from build123d import *

# Parameters (mm, degrees)
F0_W     = 100
F0_H     = 150
F1_DEPTH = 47
F2_R     = 33.5
F3_DEPTH = 22
F4_R     = 5
F5_DEPTH = 12


with BuildPart() as f1:
    # F0 (on Front) → F1 (new body)
    with BuildSketch(Plane.XZ):
        Rectangle(F0_W, F0_H)
    extrude(amount=F1_DEPTH)

    # F2 (on face) → F3 (join)
    with BuildSketch(Plane.XZ.offset(47)):
        with Locations((0, 30)):
            Circle(F2_R)
    extrude(amount=F3_DEPTH)

    # F4 (on face) → F5 (cut)
    with BuildSketch(Plane.XZ.offset(47)):
        with Locations((50, -17)):
            Circle(F4_R)
        with Locations((-50, -17)):
            Circle(F4_R)
    extrude(amount=-F5_DEPTH, mode=Mode.SUBTRACT)


solid = f1.part
The listing builds one solid part. Answer for the finished solid, in the listing's coordinates (mm). A direction names the side the tool comes from. Coordinates: 2 decimals unless noted, no trailing zeros. Write each loop counter-clockwise with the first axis right and the second up, starting at its lowest first coordinate (ties: lowest second). Pieces come first, ordered by that corner, then holes. Notation, with made-up numbers: M 78,63 L 97,63 A21 cw 97,85 Z; hole C 53.25,89.25 d6. An arc over 180 degrees is marked long. Use one line per item in the form item = value.
Item 1: Find section C-C, the plane y = -55.5. Give the vertices of the cut face in (x, z).
Model answer:
outline = C 0,30 d67
Item 2: Given P1, Ø1.5, axis at x = 46.5, z = -17.5, coming from the -Y side; P2, Ø4, axis at x = 31.5, z = -11.5, coming from the -Y side; P3, Ø10, axis at x = 34, z = -54.5, coming from the +Y side, each flat-ended and moving along its own axis, determine where each tip first touches the part or whether it passes through.
Model answer:
P1 = -35
P2 = -47
P3 = 0
Item 3: Find section A-A, the plane z = -17. Give the vertices of the cut face in (x, y), plus the area to 3 significant figures.
Model answer:
outline = M -50,-35 L -45,-35 L -45,-47 L 45,-47 L 45,-35 L 50,-35 L 50,0 L -50,0 Z
area = 4,580 mm2
Item 4: For faces 4 (the face through (48, -35, -17)), 5 (the face through (-45, -41, -17)), 6 (the face through (0, -69, 30)), 7 (the face through (50, -23, -1)), 8 (the face through (31.953, -57.846, 40.062)), determine the directions among +Z, -Z, +X, -X, +Y, -Y from which every point of the face is accessible in a straight line to the end or side of a thin tool.
Model answer:
face_4 = +X, -Y
face_5 = -X, -Y
face_6 = +Z, -Z, +X, -X, -Y
face_7 = +Z, -Z, +X, +Y, -Y
face_8 = -Y
Item 5: The mould has two halves that part along Z. Classify faces 1 (the face through (-50, -23, -1)), 2 (the face through (45, -41, -17)), 3 (the face through (-1, -23, -75)): released by +Z, released by -Z, zero draft, split by the parting line, or undercut.
Model answer:
face_1 = zero draft
face_2 = undercut
face_3 = released by -Z
Item 6: Find section B-B, the plane x = 0. Give the vertices of the cut face in (y, z), plus the area to 3 significant figures.
Model answer:
outline = M -69,-3.5 L -47,-3.5 L -47,-75 L 0,-75 L 0,75 L -47,75 L -47,63.5 L -69,63.5 Z
area = 8,520 mm2
Item 7: Find the intervals of material crossed by probe 1 along Y at (x, z) = (-2, -9); probe 2 along Z at (x, y) = (1.5, -48); probe 3 along Z at (x, y) = (18, -56), in increasing order.
Model answer:
probe_1 = -47 to 0
probe_2 = -3.47 to 63.47
probe_3 = 1.75 to 58.25
